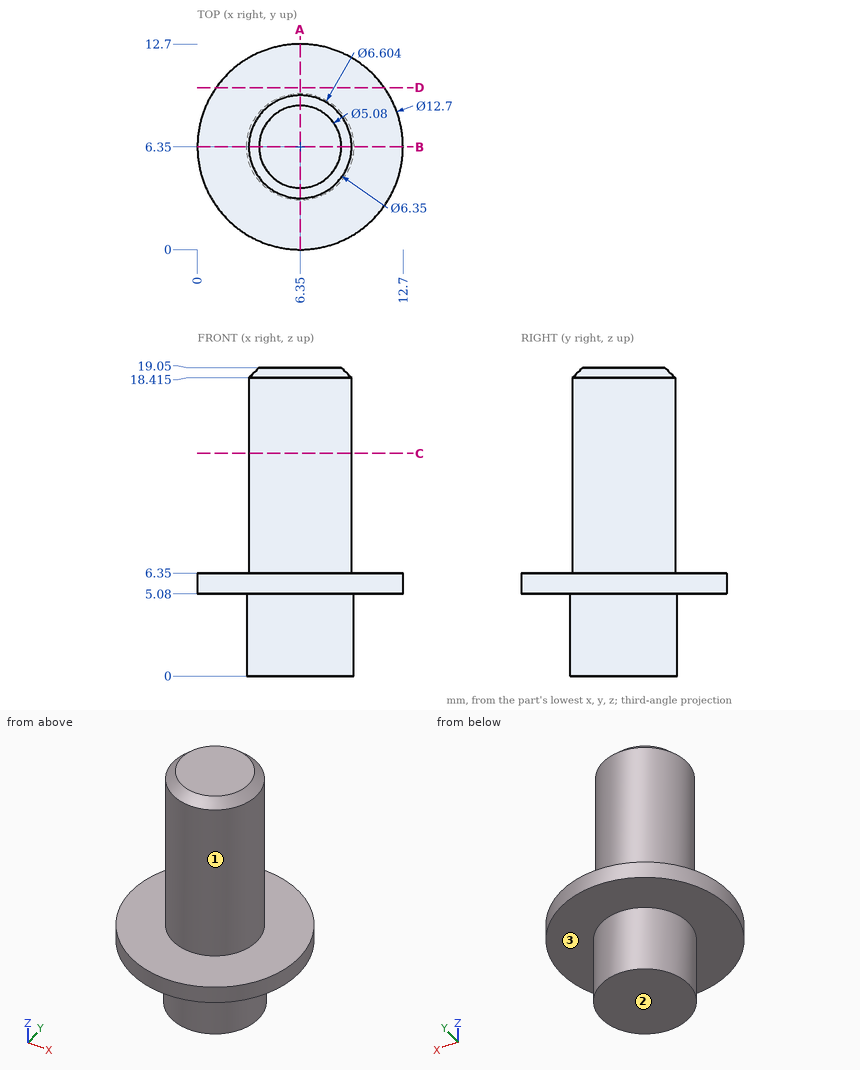
Answer from the drawing. Dimensions are ordinates in mm from the lowest x, y and z of the part. A direction names the side the tool comes from. Coordinates: 2 decimals unless noted, no trailing zeros. Order: outer loops, then holes, each group sorted by start corner. A loop starts at its lowest first (then second) coordinate and runs counter-clockwise, first axis right, second up. Notation, with made-up numbers: (-34, 54.25) - (-24, 54.25) arc R33 cw to (-24, 89.25) - close; hole circle Ø2 at (17.25, 22.25). An arc over 180 degrees is marked (long way). Use one line per item in the form item = value.
(1) Given pin 1 Ø5 at (y, z) = (8, 14) entering from +X (3 decimals); pin 2 Ø5 at (x, z) = (6.5, 10.5) entering from -Y (3 decimals); pin 3 Ø6 at (y, z) = (11, 16.5) entering from -X; pin 4 Ø4 at (x, y) = (9.5, 8.5) entering from -Z, each flat-ended and moving along its own axis, determine where each tip first touches the part or whether it passes through.
Computed values:
pin_1 = 9.525
pin_2 = 3.175
pin_3 = 3.64
pin_4 = 0
(2) Straight lines are drawn through the part: L1, parallel to Z at x = 2.75, y = 11.25; L2, parallel to Y at x = 6.5, z = 14; L3, parallel to Y at x = 3.75, z = 6.5. For each, find the intervals that lie inside material, in ascending order.
Computed values:
L1 = 5.08 to 6.35
L2 = 3.18 to 9.52
L3 = 4.53 to 8.17
(3) Section D-D, the plane y = 10 is taken. Give the vertices of the cut face in (x, z).
Computed values:
outline = (1.15, 5.08) - (11.55, 5.08) - (11.55, 6.35) - (1.15, 6.35) - close
(4) Which of the six approach directions +Z, -Z, +X, -X, +Y, -Y give full straight-line access (tool end or side, diameter ignored) to the marked faces 1, 2 and 3?
Computed values:
face_1 = +Z
face_2 = -Z, +X, -X, +Y, -Y
face_3 = -Z
(5) Section A-A, the plane x = 6.35 is taken. Give the vertices of the cut face in (y, z) (3 decimals), then the cut area to 3 significant figures.
Computed values:
outline = (0, 5.08) - (3.048, 5.08) - (3.048, 0) - (9.652, 0) - (9.652, 5.08) - (12.7, 5.08) - (12.7, 6.35) - (9.525, 6.35) - (9.525, 18.415) - (8.89, 19.05) - (3.81, 19.05) - (3.175, 18.415) - (3.175, 6.35) - (0, 6.35) - close
area = 130 mm²
(6) Section C-C, the plane z = 13.75 is taken. Give the vertices of the cut face in (x, y) (3 decimals).
Computed values:
outline = circle Ø6.35 at (6.35, 6.35)
